Geometry check sheet. Reference: the model listing, model coordinates, mm. A direction names the side the tool comes from. Coordinates: 2 decimals unless noted, no trailing zeros. Order: outer loops, then holes, each group sorted by start corner. A loop starts at its lowest first (then second) coordinate and runs counter-clockwise, first axis right, second up. Notation, with made-up numbers: M -16.75,14 L -7.75,14 A6 cw -7.75,19 Z; hole C -16.75,79 d10. An arc over 180 degrees is marked long. One line per item, written item: value. Start each with the question number.
1) Sectioned sample at B-B, the plane z = -9. Enter the section's corners in (x, y).
2) Access from +Z, -Z, +X, -X, +Y, -Y to the whole of each face (thin tool, end or side, straight path). Record for faces 1 (the flat face through (-14, -5, -0.5)), 2 (the flat face through (-17.557, -5, -6)), 3 (the flat face through (6, -5, -6.5)).
3) Draft check along X on faces 4 (the cylindrical face through (-41.101, -4.684, -18.386)), 5 (the flat face through (16.92, -4.68, -2.02)), 6 (the flat face through (-23, -9.5, -7)), 7 (the flat face through (-18, -5, -4.9)). Enter one of: pulls with the +X half, pulls with the -X half, needs draft (parallel to the pull), parting line crosses it, or undercut.
4) Sectioned sample at C-C, the plane z = -5.75. Enter the section's corners in (x, y).
5) Sectioned sample at D-D, the plane x = -8. Enter the section's corners in (y, z), then the cut area to 3 significant figures.
6) Go/stop test with flat-tipped pins: P1, Ø1, axis at x = 21.5, y = -1, coming from the -Z side; P2, Ø4, axis at y = -5.5, z = -7.5, coming from the -X side; P3, Ø3, axis at x = -34, y = -7.5, coming from the +Z side. Record where each tip stops, or that it passes through.
7) Sectioned sample at A-A, the plane y = -7. Enter the section's corners in (x, z).
8) Thickness scan on L1, parallel to X at y = -1.25, z = -5.5; L2, parallel to X at y = -4.75, z = -6; L3, parallel to X at y = -1.5, z = -7.5. Record the ranges inside material, lowest first. Write a range as from..to.
```python
from build123d import *

# Parameters (mm, degrees)
F2_DEPTH = 9.5


with BuildPart() as f2:
    # F1 (on Front) → F2 (new body)
    with BuildSketch(Plane.XZ):
        with BuildLine():
            Line((-17.5572873813, -6.5), (30.5, -6.5))
            Line((30.5, -6.5), (30.5, -3.5))
            Line((30.5, -3.5), (2.9580398915, -0.5))
            ThreePointArc((2.9580398915, -0.5), (0, -3), (-2.9580398915, -0.5))
            Line((-2.9580398915, -0.5), (-17.160677935, -0.5))
            Line((-17.160677935, -0.5), (-17.1837798887, -0.5))
            Line((-17.1837798887, -0.5), (-25, -0.5))
            ThreePointArc((-25, -0.5), (-37.6901536634, -12.7), (-50.3803073267, -0.5))
            Line((-50.3803073267, -0.5), (-56.3834679762, -0.5))
            ThreePointArc((-56.3834679762, -0.5), (-40.745644054, -18.4486850066), (-20.1561866279, -6.5))
            Line((-20.1561866279, -6.5), (-19.1572873813, -6.5))
            Line((-19.1572873813, -6.5), (-19.1572873813, -4.9))
            Line((-19.1572873813, -4.9), (-17.5572873813, -4.9))
            Line((-17.5572873813, -4.9), (-17.5572873813, -6.5))
        make_face()
    extrude(amount=F2_DEPTH)


solid = f2.part
```
Final values:
1. outline: M -54.08,-9.5 L -46.65,-9.5 L -46.65,0 L -54.08,0 Z; M -28.73,-9.5 L -21.3,-9.5 L -21.3,0 L -28.73,0 Z
2. face 1: +Z, +X, -X, +Y, -Y
2. face 2: -Z, +Y, -Y
2. face 3: -Z, +X, +Y, -Y
3. face 4: parting line crosses it
3. face 5: pulls with the +X half
3. face 6: needs draft
3. face 7: undercut
4. outline: M -55.48,-9.5 L -49.01,-9.5 L -49.01,0 L -55.48,0 Z; M -26.37,-9.5 L -19.16,-9.5 L -19.16,0 L -26.37,0 Z; M -17.56,-9.5 L 30.5,-9.5 L 30.5,0 L -17.56,0 Z
5. outline: M -9.5,-6.5 L 0,-6.5 L 0,-0.5 L -9.5,-0.5 Z
5. area: 57.0 mm^2
6. P1: stops at z = -6.5
6. P2: stops at x = -55.56
6. P3: stops at z = -11.59
7. outline: M -56.38,-0.5 A18.7 ccw -20.16,-6.5 L -19.16,-6.5 L -19.16,-4.9 L -17.56,-4.9 L -17.56,-6.5 L 30.5,-6.5 L 30.5,-3.5 L 2.96,-0.5 A3 cw -2.96,-0.5 L -25,-0.5 A12.7 cw -50.38,-0.5 Z
8. L1: x = -55.56..-49.14, -26.24..-19.16, -17.56..30.5
8. L2: x = -55.4..-48.88, -26.5..-19.16, -17.56..30.5
8. L3: x = -54.82..-47.94, -27.44..-20.56
